Build history of the part. All positions in model axes, mm. Face numbers are marked on the shaded views. A direction names the side the tool comes from. Give positions to 0.01 mm unless a question says otherwise; leave off trailing zeros. Write each loop counter-clockwise with the first axis right and the second up, starting at its lowest first coordinate (ties: lowest second). Pieces come first, ordered by that corner, then holes. Notation, with made-up numbers: (5, -20.5) - (55, -20.5) arc R11 cw to (55, -6.5) - close; hole circle Ø4 at (5.5, 3). An arc over 180 degrees is marked (long way). Use one line per item in the form item = value. Start each with the question number.
Autodesk Fusion 360 part; units mm, degrees
sketch "Sketch1" plane through (0, 0, 0) normal (0, 1, 0) x (1, 0, 0)
  line L0 (8, 0) -> (83, 0)
  line L1 (83, 0) -> (83, -8)
  line L2 (83, -8) -> (16, -8)
  line L3 (8, -16) -> (8, -89)
  line L4 (8, -89) -> (4, -89)
  line L5 (4, -89) -> (4, -83)
  line L6 (4, -83) -> (0, -83)
  line L7 (0, -83) -> (0, -8)
  arc A0 (16, -8) -> (8, -16) centre (16, -16) ccw
  arc A1 (8, 0) -> (0, -8) centre (8, -8) ccw
  line L8 (74, 0) -> (74, -4) construction
  circle A2 centre (74, -4) radius 1.5
  dimension "d1" = 83
  dimension "d2" = 8
  dimension "d3" = 4
  dimension "d4" = 8
  dimension "d5" = 8
  dimension "d6" = 8
  dimension "d7" = 89
  dimension "d8" = 83
  dimension "d9" = 75
  dimension "d11" = 4
  dimension "d12" = 3
  dimension "d13" = 66
extrude "Extrude1" add sketch "Sketch1" along normal blind 12
fillet "Fillet1" radius 6 1 edges at (6, 0, 89)
fillet "Fillet2" radius 6 1 edges at (6, 12, 89)
sketch "Sketch2" plane through (0, 0, 0) normal (1, 0, 0) x (0, 1, 0)
  arc A0 (12, 83) -> (0, 83) centre (6, 83) ccw
  line L0 (0, 83) -> (0, 16)
  line L1 (0, 16) -> (12, 16)
  line L2 (12, 16) -> (12, 83)
  line L3 (6, 16) -> (6, 83) construction
  circle A1 centre (6, 83) radius 4.5
  line L4 (0, 8) -> (0, 83)
  line L5 (0, 83) -> (12, 83)
  line L6 (12, 83) -> (12, 8)
  line L7 (12, 8) -> (0, 8)
  dimension "d20" = 67
  dimension "d21" = 9
hole "Hole1" at (0, 6, 83) direction (-1, 0, 0) diameter 9 depth 13 tip angle 118 counterbore diameter 10 counterbore depth 4
sketch "Sketch3" plane through (0, 0, 8) normal (0, 0, 1) x (-1, 0, 0)
  line L0 (-16, 0) -> (-83, 0)
  line L1 (-83, 0) -> (-83, -12)
  line L2 (-83, -12) -> (-16, -12)
  line L3 (-16, -12) -> (-16, 0)
  line L4 (-83, -6) -> (-74, -6) construction
  circle A0 centre (-74, -6) radius 3
  dimension "d27" = 9
  dimension "d28" = 6
hole "Hole2" at (74, 6, 8) direction (0, 0, -1) diameter 6 depth 13 tip angle 118
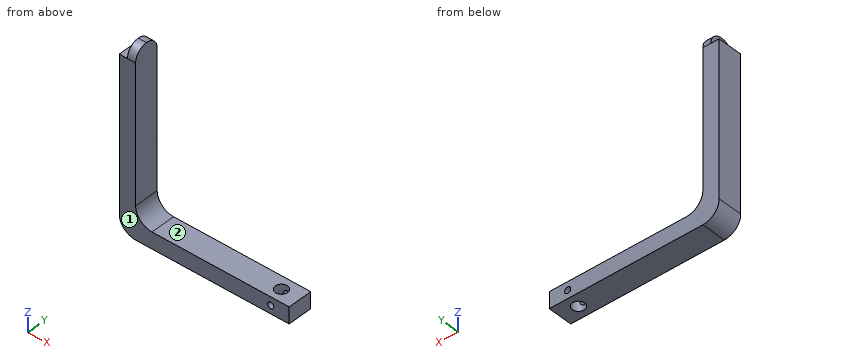
(1) Cut at D-D, the plane z = 79.5. Give the cut face in (x, y).
(2) Which spindle directions (+Z, -Z, +X, -X, +Y, -Y) get a long thin tool onto all of the face, cutting with end or side? Do the marked faces 1 and 2. Say none if no direction does.
(3) Cut at B-B, the plane z = 4. Give the cut face in (x, y).
(4) Cut at C-C, the plane x = 37. Give the cut face in (y, z), then the cut area to 3 significant figures.
(5) Wall check: line 1 (Z direction, x = 74, y = 1.6); line 2 (X direction, y = 8.5, z = 17). Give the ranges that are in metal, low to high. Write a range as from..to.
(6) Cut at A-A, the plane x = 74. Give the cut face in (y, z), then the cut area to 3 significant figures.
(7) Pin check, flat tips, straight feed: pin 1 Ø5 at (y, z) = (6, 26) entering from +X; pin 2 Ø3 at (x, y) = (17.5, 9) entering from +Z; pin 3 Ø6.5 at (y, z) = (6, 87) entering from -X. Stop position of each tip, or through.
Solution:
q1.outline = (0, 0) - (8, 0) - (8, 12) - (0, 12) - close
q2.face_1 = +Z, -Z, +X, -X, -Y
q2.face_2 = +Z, +X, +Y, -Y
q3.outline = (1.07, 0) - (72.5, 0) - (72.5, 3.4) arc R3 cw to (72.5, 8.6) - (72.5, 12) - (1.07, 12) - close; (75.5, 0) - (83, 0) - (83, 12) - (75.5, 12) - (75.5, 8.6) arc R3 cw to (75.5, 3.4) - close
q4.outline = (0, 0) - (12, 0) - (12, 8) - (0, 8) - close
q4.area = 96.0 mm2
q5.line_1 = 0..2.5, 5.5..8
q5.line_2 = 0..8
q6.outline = (0, 0) - (3, 0) - (3, 2.5) - (0, 2.5) - close; (0, 5.5) - (3, 5.5) - (3, 8) - (0, 8) - close; (9, 0) - (12, 0) - (12, 2.5) - (9, 2.5) - close; (9, 5.5) - (12, 5.5) - (12, 8) - (9, 8) - close
q6.area = 30.0 mm2
q7.pin_1 = 8
q7.pin_2 = 8
q7.pin_3 = 4
